Check sheet for the modelled part. Datum: model origin and axes. Units: mm. A direction names the side the tool comes from. Round coordinates to 2 decimals unless told otherwise and drop trailing zeros. Write each loop counter-clockwise with the first axis right and the second up, starting at its lowest first coordinate (ties: lowest second). Pieces come first, ordered by that corner, then holes. Notation, with made-up numbers: (0.5, 51.5) -> (32.5, 51.5) arc R23 ccw to (32.5, 83.5) -> close; hole circle Ø10 at (-36, -11.5). An arc over 180 degrees is marked (long way). Answer as a JSON object with one key per item and string values. Group by question number.
```python
from build123d import *

# Parameters (mm, degrees)
BOSS_EXTRUDE1_DEPTH = 61.5
CUT_EXTRUDE1_DEPTH  = 3.2
SKETCH1_5_R         = 0.9
BOSS_EXTRUDE2_DEPTH = 1.2
CUT_EXTRUDE2_START  = -3.2
SKETCH2_R           = 0.9
CUT_EXTRUDE2_DEPTH  = 3.2
BOSS_EXTRUDE3_START = -1.2
SKETCH2_4_R         = 0.9
BOSS_EXTRUDE3_DEPTH = 1.2
CUT_EXTRUDE3_DEPTH  = 3.2
BOSS_EXTRUDE4_DEPTH = 1.2
CUT_EXTRUDE4_DEPTH  = 64.798510954


with BuildPart() as part:
    # Sketch1 → Boss-Extrude1 (new body)
    with BuildSketch(Plane.XY):
        Polygon((12, 0), (0, 12), (0, 0), align=None)
    extrude(amount=BOSS_EXTRUDE1_DEPTH)

    # Sketch1_4 → Cut-Extrude1 (cut)
    with BuildSketch(Plane.XY):
        Polygon((10.535533906, 0), (4.247146227, 6.288387679), (1.458758548, 5.541241452), (0.711612321, 2.752853773), (3.464466094, 0), align=None)
    extrude(amount=CUT_EXTRUDE1_DEPTH, mode=Mode.SUBTRACT)

    # Sketch1_5 → Boss-Extrude2 (add)
    with BuildSketch(Plane.XY):
        Polygon((10.535533906, 0), (4.247146227, 6.288387679), (1.458758548, 5.541241452), (0.711612321, 2.752853773), (3.464466094, 0), align=None)
        with Locations((3.5, 3.5)):
            Circle(SKETCH1_5_R, mode=Mode.SUBTRACT)
    extrude(amount=BOSS_EXTRUDE2_DEPTH)

    # Sketch2 → Cut-Extrude2 (cut)
    with BuildSketch(Plane.XY.offset(61.5).offset(CUT_EXTRUDE2_START)):
        Polygon((2.752853773, 0.711612321), (5.541241452, 1.458758548), (6.288387679, 4.247146227), (4.247146227, 6.288387679), (1.458758548, 5.541241452), (0.711612321, 2.752853773), align=None)
        Polygon((10.535533906, 0), (6.288387679, 4.247146227), (5.541241452, 1.458758548), (2.752853773, 0.711612321), (3.464466094, 0), align=None)
        with Locations((3.5, 3.5)):
            Circle(SKETCH2_R)
    extrude(amount=CUT_EXTRUDE2_DEPTH, mode=Mode.SUBTRACT)

    # Sketch2_4 → Boss-Extrude3 (add)
    # profile 1 of 2: a face of its own
    with BuildSketch(Plane.XY.offset(61.5).offset(BOSS_EXTRUDE3_START)):
        Polygon((5.541241452, 1.458758548), (6.288387679, 4.247146227), (4.247146227, 6.288387679), (1.458758548, 5.541241452), (0.711612321, 2.752853773), (2.752853773, 0.711612321), align=None)
        with Locations((3.5, 3.5)):
            Circle(SKETCH2_4_R, mode=Mode.SUBTRACT)
    # profile 2 of 2: a face of its own
    with BuildSketch(Plane.XY.offset(61.5).offset(BOSS_EXTRUDE3_START)):
        Polygon((10.535533906, 0), (6.288387679, 4.247146227), (5.541241452, 1.458758548), (2.752853773, 0.711612321), (3.464466094, 0), align=None)
    extrude(amount=BOSS_EXTRUDE3_DEPTH)

    # Sketch4 → Cut-Extrude3 (cut)
    with BuildSketch(Plane(origin=(6, 6, 0), x_dir=(0, 0, -1), z_dir=(0.7071067811865477, 0.7071067811865475, 0))):
        with BuildLine():
            Line((-54, -1.37203272), (-51.5, 0.071342953))
            Line((-51.5, 0.071342953), (-51.5, 2.958094299))
            Line((-51.5, 2.958094299), (-54, 4.401469972))
            Line((-54, 4.401469972), (-56.5, 2.958094299))
            Line((-56.5, 2.958094299), (-56.5, 1.514718626))
            Line((-56.5, 1.514718626), (-54.9, 1.514718626))
            ThreePointArc((-54.9, 1.514718626), (-54, 2.414718626), (-53.1, 1.514718626))
            ThreePointArc((-53.1, 1.514718626), (-53.363603897, 0.878322523), (-54, 0.614718626))
            Line((-54, 0.614718626), (-54, -1.37203272))
        make_face()
        with BuildLine():
            Line((-56.5, 0.071342953), (-54, -1.37203272))
            Line((-54, -1.37203272), (-54, 0.614718626))
            ThreePointArc((-54, 0.614718626), (-54.636396103, 0.878322523), (-54.9, 1.514718626))
            Line((-54.9, 1.514718626), (-56.5, 1.514718626))
            Line((-56.5, 1.514718626), (-56.5, 0.071342953))
        make_face()
        Polygon((-56.5, -8.485281374), (-54, -8.485281374), (-54, -1.37203272), (-56.5, 0.071342953), align=None)
        with BuildLine():
            ThreePointArc((-54.9, 1.514718626), (-54.636396103, 0.878322523), (-54, 0.614718626))
            Line((-54, 0.614718626), (-54, 1.514718626))
            Line((-54, 1.514718626), (-54.9, 1.514718626))
        make_face()
        with BuildLine():
            Line((-54, 1.514718626), (-54, 0.614718626))
            ThreePointArc((-54, 0.614718626), (-53.363603897, 0.878322523), (-53.1, 1.514718626))
            ThreePointArc((-53.1, 1.514718626), (-54, 2.414718626), (-54.9, 1.514718626))
            Line((-54.9, 1.514718626), (-54, 1.514718626))
        make_face()
        Polygon((-54, -8.485281374), (-51.5, -8.485281374), (-51.5, 0.071342953), (-54, -1.37203272), align=None)
        Polygon((-7.5, -8.485281374), (-5, -8.485281374), (-5, 0.071342953), (-7.5, -1.37203272), align=None)
        Polygon((-10, -8.485281374), (-7.5, -8.485281374), (-7.5, -1.37203272), (-10, 0.071342953), align=None)
        with BuildLine():
            Line((-6.6, 1.514718626), (-5, 1.514718626))
            Line((-5, 1.514718626), (-5, 2.958094299))
            Line((-5, 2.958094299), (-7.5, 4.401469972))
            Line((-7.5, 4.401469972), (-10, 2.958094299))
            Line((-10, 2.958094299), (-10, 0.071342953))
            Line((-10, 0.071342953), (-7.5, -1.37203272))
            Line((-7.5, -1.37203272), (-7.5, 0.614718626))
            ThreePointArc((-7.5, 0.614718626), (-8.136396103, 2.151114729), (-6.6, 1.514718626))
        make_face()
        with BuildLine():
            Line((-7.5, -1.37203272), (-5, 0.071342953))
            Line((-5, 0.071342953), (-5, 1.514718626))
            Line((-5, 1.514718626), (-6.6, 1.514718626))
            ThreePointArc((-6.6, 1.514718626), (-6.863603897, 0.878322523), (-7.5, 0.614718626))
            Line((-7.5, 0.614718626), (-7.5, -1.37203272))
        make_face()
        with BuildLine():
            ThreePointArc((-7.5, 0.614718626), (-6.863603897, 0.878322523), (-6.6, 1.514718626))
            Line((-6.6, 1.514718626), (-7.5, 1.514718626))
            Line((-7.5, 1.514718626), (-7.5, 0.614718626))
        make_face()
        with BuildLine():
            Line((-7.5, 1.514718626), (-6.6, 1.514718626))
            ThreePointArc((-6.6, 1.514718626), (-8.136396103, 2.151114729), (-7.5, 0.614718626))
            Line((-7.5, 0.614718626), (-7.5, 1.514718626))
        make_face()
    extrude(amount=-CUT_EXTRUDE3_DEPTH, mode=Mode.SUBTRACT)

    # Sketch4_3 → Boss-Extrude4 (add)
    with BuildSketch(Plane(origin=(6, 6, 0), x_dir=(0, 0, -1), z_dir=(0.7071067811865477, 0.7071067811865475, 0))):
        with BuildLine():
            Line((-54, -1.37203272), (-51.5, 0.071342953))
            Line((-51.5, 0.071342953), (-51.5, 2.958094299))
            Line((-51.5, 2.958094299), (-54, 4.401469972))
            Line((-54, 4.401469972), (-56.5, 2.958094299))
            Line((-56.5, 2.958094299), (-56.5, 1.514718626))
            Line((-56.5, 1.514718626), (-54.9, 1.514718626))
            ThreePointArc((-54.9, 1.514718626), (-54, 2.414718626), (-53.1, 1.514718626))
            ThreePointArc((-53.1, 1.514718626), (-53.363603897, 0.878322523), (-54, 0.614718626))
            Line((-54, 0.614718626), (-54, -1.37203272))
        make_face()
        with BuildLine():
            Line((-56.5, 0.071342953), (-54, -1.37203272))
            Line((-54, -1.37203272), (-54, 0.614718626))
            ThreePointArc((-54, 0.614718626), (-54.636396103, 0.878322523), (-54.9, 1.514718626))
            Line((-54.9, 1.514718626), (-56.5, 1.514718626))
            Line((-56.5, 1.514718626), (-56.5, 0.071342953))
        make_face()
        Polygon((-54, -8.485281374), (-51.5, -8.485281374), (-51.5, 0.071342953), (-54, -1.37203272), align=None)
        Polygon((-56.5, -8.485281374), (-54, -8.485281374), (-54, -1.37203272), (-56.5, 0.071342953), align=None)
        with BuildLine():
            Line((-6.6, 1.514718626), (-5, 1.514718626))
            Line((-5, 1.514718626), (-5, 2.958094299))
            Line((-5, 2.958094299), (-7.5, 4.401469972))
            Line((-7.5, 4.401469972), (-10, 2.958094299))
            Line((-10, 2.958094299), (-10, 0.071342953))
            Line((-10, 0.071342953), (-7.5, -1.37203272))
            Line((-7.5, -1.37203272), (-7.5, 0.614718626))
            ThreePointArc((-7.5, 0.614718626), (-8.136396103, 2.151114729), (-6.6, 1.514718626))
        make_face()
        with BuildLine():
            Line((-7.5, -1.37203272), (-5, 0.071342953))
            Line((-5, 0.071342953), (-5, 1.514718626))
            Line((-5, 1.514718626), (-6.6, 1.514718626))
            ThreePointArc((-6.6, 1.514718626), (-6.863603897, 0.878322523), (-7.5, 0.614718626))
            Line((-7.5, 0.614718626), (-7.5, -1.37203272))
        make_face()
        Polygon((-7.5, -8.485281374), (-5, -8.485281374), (-5, 0.071342953), (-7.5, -1.37203272), align=None)
        Polygon((-10, -8.485281374), (-7.5, -8.485281374), (-7.5, -1.37203272), (-10, 0.071342953), align=None)
    extrude(amount=-BOSS_EXTRUDE4_DEPTH)

    # Sketch1_6 → Cut-Extrude4 (cut, through all)
    with BuildSketch(Plane.XY):
        Polygon((12, -2.237434652), (12, 0), (10.535533906, 0), (7, 0), (3.5, 0), (3.464466094, 0), (0, 0), (0, -2.237434652), align=None)
    extrude(amount=CUT_EXTRUDE4_DEPTH, mode=Mode.SUBTRACT)


solid = part.part
```
(1) Section check B-B on x = 9.5. Record the cut outline in (y, z).
(2) Go/stop test with flat-tipped pins: pin 1 Ø1.6 at (x, y) = (3.5, 3.5) entering from -Z; pin 2 Ø1.6 at (x, y) = (3.5, 3.5) entering from +Z; pin 3 Ø4 at (x, y) = (8, 7) entering from -Z; pin 4 Ø3 at (y, z) = (10, 35) entering from +X. Record where each tip stops, or that it passes through.
(3) Section check D-D on y = 9.5. Record the cut outline in (x, z).
(4) Access from +Z, -Z, +X, -X, +Y, -Y to the whole of each face (thin tool, end or side, straight path). Record for faces 1 (the flat face through (7.435, 3.1, 2.186)), 2 (the cylindrical face through (3.305, 2.621, 60.892)), 3 (the flat face through (6, 3, 10)).
(5) Section check C-C on z = 36.5. Record the cut outline in (x, y).
(6) Section check A-A on y = 3.5. Record the cut outline in (x, z), then the cut area to 3 significant figures.
(7) Release check for a two-part mould opening along Y. For faces 4 (the flat face through (4.002, 3.473, 7.535)), 5 (the flat face through (7.435, 3.1, 59.286)), 6 (the flat face through (0, 6, 30)), 7 (the flat face through (4, 2, 58.3)) record: pulls with the +Y half, pulls with the -Y half, needs draft (parallel to the pull), parting line crosses it, or undercut.
(8) Scan lines: line 1 along Z through (x, y) = (5.25, 2); line 2 along Z through (x, y) = (7, 1.5); line 3 along Y through (x, z) = (3.5, 0.75). Record each from-to range of solid material in increasing order.
Data:
{
 "1": {"outline": "(0, 0) -> (2.5, 0) -> (2.5, 61.5) -> (0, 61.5) -> (0, 60.3) -> (1.04, 60.3) -> (1.04, 58.3) -> (0, 58.3) -> (0, 56.5) -> (0.8, 56.5) -> (0.8, 51.5) -> (0, 51.5) -> (0, 10) -> (0.8, 10) -> (0.8, 5) -> (0, 5) -> (0, 3.2) -> (1.04, 3.2) -> (1.04, 1.2) -> (0, 1.2) -> close"},
 "2": {"pin 1": "stops at z = 3.2", "pin 2": "stops at z = 58.3", "pin 3": "passes through", "pin 4": "stops at x = 3.5"},
 "3": {"outline": "(0, 0) -> (2.5, 0) -> (2.5, 61.5) -> (0, 61.5) -> close"},
 "4": {"face 1": "-Y", "face 2": "+Z", "face 3": "none"},
 "5": {"outline": "(0, 0) -> (12, 0) -> (0, 12) -> close"},
 "6": {"outline": "(0, 0) -> (2.6, 0) -> (2.6, 1.2) -> (0.91, 1.2) -> (0.91, 3.2) -> (7.04, 3.2) -> (7.04, 1.2) -> (4.4, 1.2) -> (4.4, 0) -> (8.5, 0) -> (8.5, 61.5) -> (4.4, 61.5) -> (4.4, 60.3) -> (7.04, 60.3) -> (7.04, 58.3) -> (0.91, 58.3) -> (0.91, 60.3) -> (2.6, 60.3) -> (2.6, 61.5) -> (0, 61.5) -> close; hole (3.97, 5) -> (6.8, 5) -> (6.8, 10) -> (3.97, 10) -> close; hole (3.97, 51.5) -> (6.8, 51.5) -> (6.8, 56.5) -> (3.97, 56.5) -> close", "area": "466 mm²"},
 "7": {"face 4": "undercut", "face 5": "pulls with the -Y half", "face 6": "needs draft", "face 7": "undercut"},
 "8": {"line 1": "z = 0 to 1.2, 3.2 to 58.3, 60.3 to 61.5", "line 2": "z = 0 to 1.2, 3.2 to 5, 10 to 51.5, 56.5 to 58.3, 60.3 to 61.5", "line 3": "y = 0 to 2.6, 4.4 to 8.5"}
}
